Design review of the part built by this model. Coordinates are the model's own, in mm. Face numbers are marked on the shaded views. A direction names the side the tool comes from. Coordinates: 2 decimals unless noted, no trailing zeros. Loops run counter-clockwise (first coordinate to the right, second up) from the corner with the lowest first, then second, coordinate; pieces in that order, holes last. Notation, with made-up numbers: M -10,32.25 L 14,32.25 A33 ccw 14,60.25 Z; hole C 79,-14.5 d10. An arc over 180 degrees is marked long. Answer as a JSON object with one key per item and string values. Group by question number.
1. To check wall thickness, follow probe 1 along X at (y, z) = (1.35, -0.05); probe 2 along Y at (x, z) = (-0.5, 0); probe 3 along Y at (x, z) = (-2, -0.5). State the ranges of each line that lie inside material, in increasing order.
2. Consider section A-A (z = 4.5). State the section outline as (x, y) points, then the cut area to 3 significant figures.
3. Insertion check: pin 1 (1.5 mm diameter, centred on x = 2, y = 0.5, fed in from -Z); pin 2 (4 mm diameter, centred on x = 0, z = -0.5, fed in from +Y); pin 3 (1.5 mm diameter, centred on x = 0.5, y = 3, fed in from +Z). Each pin has a flat end and moves straight along its axis. Give the tip position at first contact, or say it passes through.
4. Consider section D-D (z = -0.05). State the section outline as (x, y) points.
5. Draft analysis for pull direction Z (two halves, no side actions). For the marked faces 1, 2 and 3, state which applies: +Z half, -Z half, draft (parallel to the pull), parting line (faces both ways), or undercut.
6. Machinability: for the marked faces 4, 5, 6 and 7, which of the approach directions +Z, -Z, +X, -X, +Y, -Y give a long, thin tool a straight path to every point of the face, cutting with its end or side? Answer none if there is none.
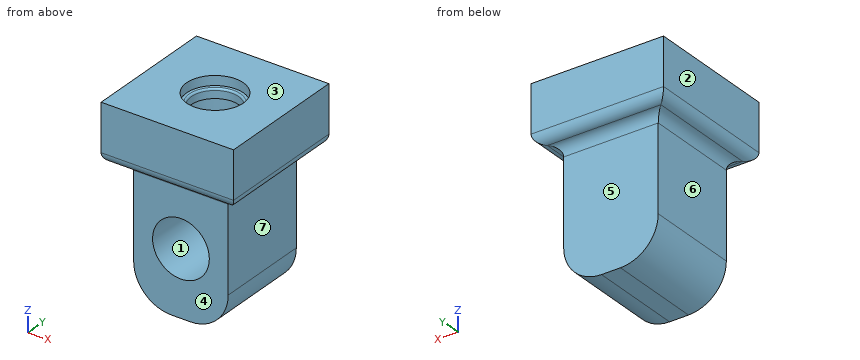
from build123d import *

# Parameters (mm, degrees)
ESQUISSE4_R             = 1.5
BOSS_EXTRU_2_DEPTH      = 5
BOSS_EXTRU_3_START      = -2
ESQUISSE5_R             = 1.5
BOSS_EXTRU_3_DEPTH      = 2
ESQUISSE6_W             = 7
ESQUISSE6_H             = 7
BOSS_EXTRU_4_DEPTH      = 3
CONG_1_R                = 0.5
ESQUISSE7_R             = 1.5
ENL_V_MAT_EXTRU_1_DEPTH = 3
BOSS_EXTRU_5_START      = -0.5
ESQUISSE8_R             = 1.5
ESQUISSE8_R_2           = 1.25
BOSS_EXTRU_5_DEPTH      = 0.5
CONG_2_R                = 0.1


with BuildPart() as part:
    # Esquisse4 → Boss.-Extru.2 (new body)
    with BuildSketch(Plane(origin=(0, 0, 0), x_dir=(1, 0, 0), z_dir=(0, 1, 0))):
        with BuildLine():
            Line((-0.5, 3.5), (0.5, 3.5))
            ThreePointArc((0.5, 3.5), (1.914213562, 2.914213562), (2.5, 1.5))
            Line((2.5, 1.5), (2.5, -3.5))
            Line((2.5, -3.5), (-2.5, -3.5))
            Line((-2.5, -3.5), (-2.5, 1.5))
            ThreePointArc((-2.5, 1.5), (-1.914213562, 2.914213562), (-0.5, 3.5))
        make_face()
        with Locations(Location((0, 0.05, 0), (0, 0, 270))):
            Circle(ESQUISSE4_R, mode=Mode.SUBTRACT)
    extrude(amount=BOSS_EXTRU_2_DEPTH)

    # Esquisse5 → Boss.-Extru.3 (add)
    with BuildSketch(Plane(origin=(0, 5, 0), x_dir=(1, 0, 0), z_dir=(0, 1, 0)).offset(BOSS_EXTRU_3_START)):
        with Locations(Location((0, 0.05, 0), (0, 0, 270))):
            Circle(ESQUISSE5_R)
    extrude(amount=BOSS_EXTRU_3_DEPTH)

    # Esquisse6 → Boss.-Extru.4 (add)
    with BuildSketch(Plane.XY.offset(3.5)):
        with Locations((0, 2.5)):
            Rectangle(ESQUISSE6_W, ESQUISSE6_H)
    extrude(amount=BOSS_EXTRU_4_DEPTH)

    # Congé1
    cong_1_edges = [part.edges().sort_by_distance(p)[0] for p in [
        (2.5, 2.5, 3.5),
        (-2.5, 2.5, 3.5),
        (0, 5, 3.5),
        (-3.5, 2.5, 3.5),
        (0, -1, 3.5),
        (3.5, 2.5, 3.5),
        (0, 6, 3.5),
        (0, 0, 3.5),
    ]]
    fillet(cong_1_edges, radius=CONG_1_R - 0.0001)  # a hair under: the kernel refuses the full size

    # Esquisse7 → Enlèv. mat.-Extru.1 (cut)
    with BuildSketch(Plane.XY.offset(6.5)):
        with Locations((0, 2.5)):
            Circle(ESQUISSE7_R)
    extrude(amount=-ENL_V_MAT_EXTRU_1_DEPTH, mode=Mode.SUBTRACT)

    # Esquisse8 → Boss.-Extru.5 (add)
    with BuildSketch(Plane.XY.offset(6.5).offset(BOSS_EXTRU_5_START)):
        with Locations((0, 2.5)):
            Circle(ESQUISSE8_R)
        with Locations((0, 2.5)):
            Circle(ESQUISSE8_R_2, mode=Mode.SUBTRACT)
    extrude(amount=-BOSS_EXTRU_5_DEPTH)

    # Congé2
    cong_2_edges = [part.edges().sort_by_distance(p)[0] for p in [
        (-1.25, 2.5, 6),
    ]]
    fillet(cong_2_edges, radius=CONG_2_R)


solid = part.part
Findings below:
{
 "1": {"probe 1": "x = -2.5 to -1.5, 1.5 to 2.5", "probe 2": "y = 3 to 5", "probe 3": "y = 0 to 5"},
 "2": {"outline": "M -3.5,-1 L 3.5,-1 L 3.5,6 L -3.5,6 Z; hole C 0,2.5 d3", "area": "41.9 mm^2"},
 "3": {"pin 1": "stops at z = -3.35", "pin 2": "stops at y = 5", "pin 3": "stops at z = 6"},
 "4": {"outline": "M -2.5,0 L -1.5,0 L -1.5,3 L 1.5,3 L 1.5,0 L 2.5,0 L 2.5,5 L -2.5,5 Z"},
 "5": {"face 1": "undercut", "face 2": "draft", "face 3": "+Z half"},
 "6": {"face 4": "-Z, +X, -X, -Y", "face 5": "-Z, +X, -X, +Y", "face 6": "-Z, -X, +Y, -Y", "face 7": "-Z, +X, +Y, -Y"}
}
